Part model, mm, in its own coordinate system. Face numbers are marked on the shaded views. Round coordinates to 2 decimals unless told otherwise and drop trailing zeros. Write each loop counter-clockwise with the first axis right and the second up, starting at its lowest first coordinate (ties: lowest second). Pieces come first, ordered by that corner, then holes. Notation, with made-up numbers: M 23,62.5 L 34,62.5 A21 cw 34,100.5 Z; hole C 1,29.25 d4. An arc over 180 degrees is marked long. Use one line per item in the form item = value. Start each with the question number.
Item 1: Cut at C-C, the plane x = -38. Give the cut face in (y, z).
Item 2: Cut at A-A, the plane y = 33. Give the cut face in (x, z).
Item 3: Flat gauge pin, fed straight in: pin 1 Ø6.5 at (x, y) = (38, 53) entering from +Z. Where does the tip first touch, or does it go through?
Item 4: Mould opens along Y. For the marked faces 1 and 2 say: +Y half, -Y half, draft (parallel to the pull), parting line (faces both ways), or undercut.
Item 5: Cut at D-D, the plane x = 33.5. Give the cut face in (y, z).
Item 6: Probe L1, parallel to Y at x = -38, z = 3.1; L2, parallel to Y at x = -3, z = 3.25; L3, parallel to Z at x = -9, y = -20. List the from-to ranges inside material, lowest first.
from build123d import *

# Parameters (mm, degrees)
SKIZZE1_W                       = 100
SKIZZE1_H                       = 130
AUFSATZ_LINEAR_AUSTRAGEN1_DEPTH = 5
SKIZZE2_R                       = 30
SKIZZE2_R_2                     = 27
AUFSATZ_LINEAR_AUSTRAGEN2_DEPTH = 3
SKIZZE4_R                       = 2.5
SKIZZE4_W                       = 50
SKIZZE4_H                       = 5
SCHNITT_LINEAR_AUSTRAGEN1_DEPTH = 83.158383626
FASE1_SIZE2                     = 3
FASE1_SIZE                      = 1
VERRUNDUNG1_R                   = 5


with BuildPart() as part:
    # Skizze1 → Aufsatz-Linear austragen1 (new body)
    with BuildSketch(Plane.XY):
        Rectangle(SKIZZE1_W, SKIZZE1_H)
    extrude(amount=AUFSATZ_LINEAR_AUSTRAGEN1_DEPTH)

    # Skizze2 → Aufsatz-Linear austragen2 (add)
    with BuildSketch(Plane.XY.offset(5)):
        with Locations(Location((0, -30, 0), (0, 0, 180))):
            Circle(SKIZZE2_R)
        with Locations((0, -30)):
            Circle(SKIZZE2_R_2, mode=Mode.SUBTRACT)
    extrude(amount=AUFSATZ_LINEAR_AUSTRAGEN2_DEPTH)

    # Skizze4 → Schnitt-Linear austragen1 (cut, through all)
    with BuildSketch(Plane.XY.offset(5)):
        with Locations((-38, -53)):
            Circle(SKIZZE4_R)
        with Locations((38, -53)):
            Circle(SKIZZE4_R)
        with Locations((38, 53)):
            Circle(SKIZZE4_R)
        with Locations((-38, 53)):
            Circle(SKIZZE4_R)
        with Locations((-38, -33)):
            Circle(SKIZZE4_R)
        with Locations((38, -33)):
            Circle(SKIZZE4_R)
        with Locations((38, 33)):
            Circle(SKIZZE4_R)
        with Locations((-38, 33)):
            Circle(SKIZZE4_R)
        with Locations((0, 7.5)):
            Rectangle(SKIZZE4_W, SKIZZE4_H)
    extrude(amount=-SCHNITT_LINEAR_AUSTRAGEN1_DEPTH, mode=Mode.SUBTRACT)

    # Fase1
    fase1_edges = [part.edges().sort_by_distance(p)[0] for p in [
        (-27, -30, 8),
    ]]
    fase1_side = [part.faces().sort_by_distance(p)[0] for p in [
        (-27.02, -30, 8),
    ]]
    chamfer(fase1_edges, length=FASE1_SIZE - 0.0001, length2=FASE1_SIZE2 - 0.0001, reference=fase1_side[0])  # a hair under: the kernel refuses the full size

    # Verrundung1
    verrundung1_edges = [part.edges().sort_by_distance(p)[0] for p in [
        (50, -65, 2.5),
        (-50, -65, 2.5),
        (-50, 65, 2.5),
        (50, 65, 2.5),
    ]]
    fillet(verrundung1_edges, radius=VERRUNDUNG1_R)


solid = part.part
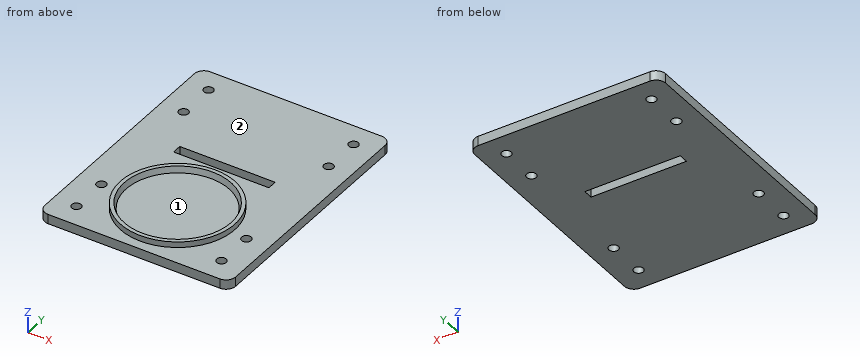
Model answer:
q1.outline = M -65,0 L -55.5,0 L -55.5,5 L -65,5 Z; M -50.5,0 L -35.5,0 L -35.5,5 L -50.5,5 Z; M -30.5,0 L 30.5,0 L 30.5,5 L -30.5,5 Z; M 35.5,0 L 50.5,0 L 50.5,5 L 35.5,5 Z; M 55.5,0 L 65,0 L 65,5 L 55.5,5 Z
q2.outline = M -50,0 L -40.5,0 L -40.5,5 L -50,5 Z; M -35.5,0 L 35.5,0 L 35.5,5 L -35.5,5 Z; M 40.5,0 L 50,0 L 50,5 L 40.5,5 Z
q3.pin_1 = 5
q4.face_1 = undercut
q4.face_2 = draft
q5.outline = M -65,0 L 65,0 L 65,5 L -65,5 Z
q6.L1 = -65 to -55.5, -50.5 to -35.5, -30.5 to 30.5, 35.5 to 50.5, 55.5 to 65
q6.L2 = -65 to 5, 10 to 65
q6.L3 = 0 to 5
